Here's how the part is built. I have some questions about the finished solid (model axes, mm). Face numbers are marked on the shaded views. A direction names the side the tool comes from. Round coordinates to 2 decimals unless told otherwise and drop trailing zeros. Write each loop counter-clockwise with the first axis right and the second up, starting at its lowest first coordinate (ties: lowest second). Pieces come first, ordered by that corner, then holes. Notation, with made-up numbers: (32, 82) -> (77, 82) arc R13 ccw to (77, 94) -> close; hole circle Ø10 at (85, 65.5). An arc over 180 degrees is marked (long way). Answer as CSV lines item,"result".
from build123d import *

# Parameters (mm, degrees)
BASE_FLANGE1_DEPTH = 75
SKETCH6_R          = 4.5
CUT_EXTRUDE1_DEPTH = 160.590099944


# Sheet-metal steps are written as plain solids
with BuildPart() as part:
    # Sketch1 → Base-Flange1 (new body)
    with BuildSketch(Plane.XY):
        with BuildLine():
            Line((0, 0), (0, 99.75))
            ThreePointArc((0, 99.75), (-0.073223305, 99.926776695), (-0.25, 100))
            Line((-0.25, 100), (-78, 100))
            Line((-78, 100), (-78, 110))
            Line((-78, 110), (-0.25, 110))
            ThreePointArc((-0.25, 110), (6.997844507, 106.997844507), (10, 99.75))
            Line((10, 99.75), (10, 0))
            Line((10, 0), (0, 0))
        make_face()
    extrude(amount=BASE_FLANGE1_DEPTH)

    # Sketch6 → Cut-Extrude1 (cut, through all)
    with BuildSketch(Plane(origin=(10, 0, 0), x_dir=(0, 0, -1), z_dir=(1, 0, 0))):
        with Locations((-60, 18)):
            Circle(SKETCH6_R)
        with Locations((-15, 18)):
            Circle(SKETCH6_R)
        with Locations((-60, 68)):
            Circle(SKETCH6_R)
        with Locations((-15, 68)):
            Circle(SKETCH6_R)
    extrude(amount=-CUT_EXTRUDE1_DEPTH, mode=Mode.SUBTRACT)


solid = part.part
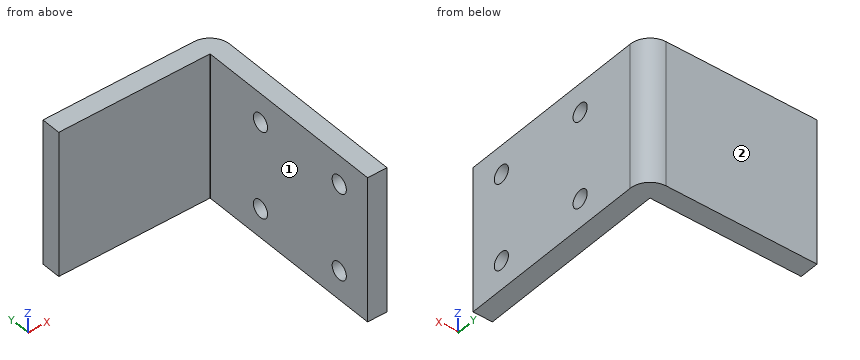
Item 1: I need wall thicknesses on L1, parallel to Y at x = 2.75, z = 60; L2, parallel to Y at x = 4.5, z = 15; L3, parallel to Y at x = -5, z = 49.5. Which ranges of each line are inside material? Lowest first, please.
Results found:
L1,"y = 0 to 13.5, 22.5 to 63.5, 72.5 to 109.55"
L2,"y = 0 to 13.5, 22.5 to 63.5, 72.5 to 108.83"
L3,"y = 100 to 110"
Item 2: For the marked faces 1 and 2, which set-ups out of +Z, -Z, +X, -X, +Y, -Y let a thin tool reach every point of the face, with its end or its side?
Results found:
face 1,"+Z, -Z, -X, -Y"
face 2,"+Z, -Z, +X, -X, +Y"
Item 3: Suppose I cut it at C-C, the plane z = 67.5. List the corners of the cut face in (x, y) for me, then the cut area to 3 significant figures.
Results found:
outline,"(-78, 100) -> (-0.25, 100) arc R0.25 cw to (0, 99.75) -> (0, 0) -> (10, 0) -> (10, 99.75) arc R10.25 ccw to (-0.25, 110) -> (-78, 110) -> close"
area,"1,860 mm²"
Item 4: Suppose I cut it at B-B, the plane z = 15. List the corners of the cut face in (x, y) for me.
Results found:
outline,"(-78, 100) -> (-0.25, 100) arc R0.25 cw to (0, 99.75) -> (0, 72.5) -> (10, 72.5) -> (10, 99.75) arc R10.25 ccw to (-0.25, 110) -> (-78, 110) -> close; (0, 0) -> (10, 0) -> (10, 13.5) -> (0, 13.5) -> close; (0, 22.5) -> (10, 22.5) -> (10, 63.5) -> (0, 63.5) -> close"
Item 5: Suppose I cut it at D-D, the plane x = -36.5. List the corners of the cut face in (y, z) for me.
Results found:
outline,"(100, 0) -> (110, 0) -> (110, 75) -> (100, 75) -> close"
Item 6: Will these pins go through, and if not, where does the flat tip stop? pin 1 (14.5 mm diameter, centred on y = 18, z = 15, fed in from +X); pin 2 (8 mm diameter, centred on y = 68, z = 15, fed in from +X); pin 3 (1.5 mm diameter, centred on x = -46, z = 60, fed in from -Y); pin 4 (11.5 mm diameter, centred on y = 68, z = 60, fed in from -X).
Results found:
pin 1,"stops at x = 10"
pin 2,"passes through"
pin 3,"stops at y = 100"
pin 4,"stops at x = 0"
Item 7: Suppose I cut it at A-A, the plane y = 18. List the corners of the cut face in (x, z) for me, then the cut area to 3 significant figures.
Results found:
outline,"(0, 0) -> (10, 0) -> (10, 10.5) -> (0, 10.5) -> close; (0, 19.5) -> (10, 19.5) -> (10, 55.5) -> (0, 55.5) -> close; (0, 64.5) -> (10, 64.5) -> (10, 75) -> (0, 75) -> close"
area,"570 mm²"
